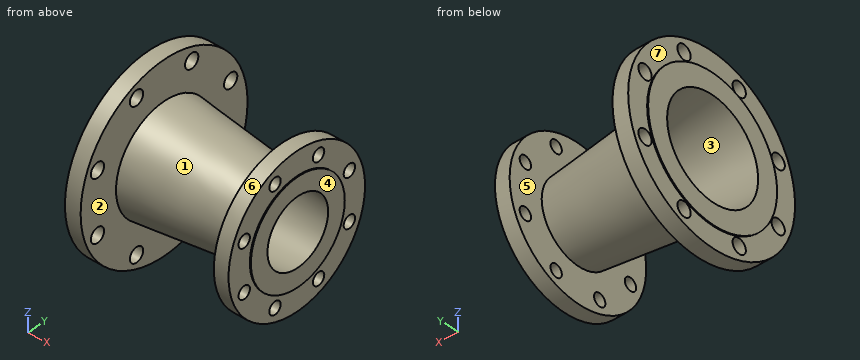
Autodesk Inventor part; units mm, degrees
ref_plane "YZ Plane" through (0, 0, 0) normal (1, 0, 0) x (0, 1, 0)
ref_plane "XZ Plane" through (0, 0, 0) normal (0, 1, 0) x (-1, 0, 0)
ref_plane "XY Plane" through (0, 0, 0) normal (0, 0, 1) x (1, 0, 0)
sketch "Sketch1" plane through (0, 0, 0) normal (0, 0, 1) x (1, 0, 0)
  line L0 (0, 0) -> (228.6, 0) construction
  line L1 (228.6, 0) -> (228.6, 50.8) construction
  line L2 (228.6, 78.613) -> (227.076, 78.613)
  line L3 (227.076, 78.613) -> (227.076, 114.3)
  line L4 (227.076, 114.3) -> (204.724, 114.3)
  line L5 (204.724, 114.3) -> (204.724, 60.6087)
  line L6 (204.724, 60.6087) -> (25.4, 80.5335)
  line L7 (25.4, 80.5335) -> (25.4, 139.7)
  line L8 (25.4, 139.7) -> (1.524, 139.7)
  line L9 (1.524, 139.7) -> (1.524, 107.95)
  line L10 (1.524, 107.95) -> (0, 107.95)
  line L11 (0, 107.95) -> (0, 76.2)
  line L12 (0, 76.2) -> (228.6, 50.8)
  line L13 (0, 76.2) -> (0, 0) construction
  line L14 (228.6, 78.613) -> (228.6, 50.8)
  dimension "d0" = 1.524
  dimension "d3" = 1.524
  dimension "d4" = 152.4
  dimension "d5" = 7.112
  dimension "d6" = 101.6
  dimension "d7" = 215.9
  dimension "d8" = 157.226
  dimension "d9" = 279.4
  dimension "d10" = 228.6
  dimension "d11" = 228.6
  dimension "d12" = 25.4
  dimension "d13" = 23.876
revolve "Revolution1" add sketch "Sketch1" angle 360 about axis through (0, 0, 0) along (1, 0, 0)
sketch "Sketch3" plane through (1.524, 0, 0) normal (-1, 0, 0) x (0, 0, 1)
  circle A0 centre (0, 0) radius 107.95
  circle A1 centre (46.1708, 111.4661) radius 11.1125
  circle A2 centre (0, 0) radius 120.65 construction
  line L0 (46.1708, 111.4661) -> (0, 0) construction
  line L1 (0, 0) -> (0, 120.65) construction
  dimension "d19" = 22.5
  dimension "d20" = 22.225
  dimension "d21" = 241.3
extrude "Extrusion1" cut sketch "Sketch3" against normal up to surface (23.876 mm away) contours A1
pattern_circular "Circular Pattern1" count 8 over 360 about axis through (13.462, 0, 0) along (1, 0, 0) of "Extrusion1"
sketch "Sketch4" plane through (227.076, 0, 0) normal (1, 0, 0) x (0, 0, -1)
  circle A0 centre (0, 0) radius 114.3
  circle A1 centre (-87.9995, 36.4506) radius 9.525
  circle A2 centre (0, 0) radius 95.25 construction
  line L0 (-87.9995, 36.4506) -> (0, 0) construction
  line L1 (0, 0) -> (-95.25, 0) construction
  dimension "d24" = 22.5
  dimension "d26" = 19.05
  dimension "d27" = 190.5
extrude "Extrusion2" cut sketch "Sketch4" against normal up to surface (22.352 mm away) contours A1
pattern_circular "Circular Pattern2" count 8 over 360 about axis through (215.9, 0, 0) along (1, 0, 0) of "Extrusion2"
equation "\"d4\" = d1"
equation "\"d5\" = t"
equation "\"d6\" = d2"
equation "\"d7\" = R1"
equation "\"d8\" = R2"
equation "\"d9\" = O1"
equation "\"d10\" = O2"
equation "\"d11\" = GG"
equation "\"d12\" = C11"
equation "\"d13\" = C12"
equation "\"d20\" = DH1"
equation "\"d21\" = BC1"
equation "\"d26\" = DH2"
equation "\"d27\" = BC2"
equation "\"O1\" = 279.4"
equation "\"C11\" = 25.4"
equation "\"t\" = 7.112"
equation "\"d1\" = 152.4"
equation "\"GG\" = 228.6"
equation "\"R1\" = 215.9"
equation "\"BC1\" = 241.3"
equation "\"DH1\" = 22.225"
equation "\"O2\" = 228.6"
equation "\"C12\" = 23.876"
equation "\"d2\" = 101.6"
equation "\"R2\" = 157.226"
equation "\"BC2\" = 190.5"
equation "\"DH2\" = 19.05"
equation "\"Size_Designation\" = 1.2345"
properties part number "ADREF-000036" material "Steel, Mild"
Here's how the part is built. I have some questions about the finished solid (model axes, mm). Face numbers are marked on the shaded views. A direction names the side the tool comes from. Give positions to 0.01 mm unless a question says otherwise; leave off trailing zeros. Loops run counter-clockwise (first coordinate to the right, second up) from the corner with the lowest first, then second, coordinate; pieces in that order, holes last. Notation, with made-up numbers: M 4,-18 L 62,-18 A25 cw 62,8 Z; hole C -8.75,35.5 d7. An arc over 180 degrees is marked long. Put each result on its own line as item: value. Start each with the question number.
(1) For the marked faces 5, 6 and 7, which set-ups out of +Z, -Z, +X, -X, +Y, -Y let a thin tool reach every point of the face, with its end or its side?
(2) I want a section at D-D on x = 112.5. Please give me the cut outline in (y, z), then the cut area to 3 significant figures.
(3) I want a section at A-A on z = 0. Please give me the cut outline in (x, y), then the cut area to 3 significant figures.
(4) I need wall thicknesses on line 1 along X through (y, z) = (86, -11); line 2 along Z through (x, y) = (208.5, -37.5); line 3 along X through (y, z) = (62.5, 94.5). Which ranges of each line are inside material? Lowest first, please. Write a range as [from, to].
(5) If we mould it in two halves opening along X, with no side actions, what happens to the marked faces 1, 2, 3 and 4? For each: +X half, -X half, draft (parallel to the pull), parting line (faces both ways), or undercut.
(6) Will these pins go through, and if not, where does the flat tip stop? pin 1 Ø4 at (x, y) = (183.5, 57.5) entering from +Z; pin 2 Ø10 at (x, z) = (113.5, 25) entering from +Y; pin 3 Ø18 at (y, z) = (-46.17, -111.47) entering from +X; pin 4 Ø22 at (y, z) = (-88, 36.45) entering from -X.
(7) I want a section at C-C on x = 41. Please give me the cut outline in (y, z), then the cut area to 3 significant figures.
Answer block:
1. face 5: none
1. face 6: +X
1. face 7: -X
2. outline: C 0,0 d141.71; hole C 0,0 d127.4
2. area: 3,020 mm^2
3. outline: M 0,-107.95 L 1.52,-107.95 L 1.52,-139.7 L 25.4,-139.7 L 25.4,-80.53 L 204.72,-60.61 L 204.72,-114.3 L 227.08,-114.3 L 227.08,-78.61 L 228.6,-78.61 L 228.6,-50.8 L 0,-76.2 Z; M 0,76.2 L 228.6,50.8 L 228.6,78.61 L 227.08,78.61 L 227.08,114.3 L 204.72,114.3 L 204.72,60.61 L 25.4,80.53 L 25.4,139.7 L 1.52,139.7 L 1.52,107.95 L 0,107.95 Z
3. area: 8,630 mm^2
4. line 1: [0, 25.4], [204.72, 227.08]
4. line 2: [-107.97, -97.47], [-78.53, -37.5], [37.5, 78.53], [97.47, 107.97]
4. line 3: [1.52, 25.4], [204.72, 227.08]
5. face 1: undercut
5. face 2: undercut
5. face 3: -X half
5. face 4: +X half
6. pin 1: z = 29.77
6. pin 2: y = 67.97
6. pin 3: x = 227.08
6. pin 4: x = 0
7. outline: C 0,0 d157.6; hole C 0,0 d143.29
7. area: 3,380 mm^2
